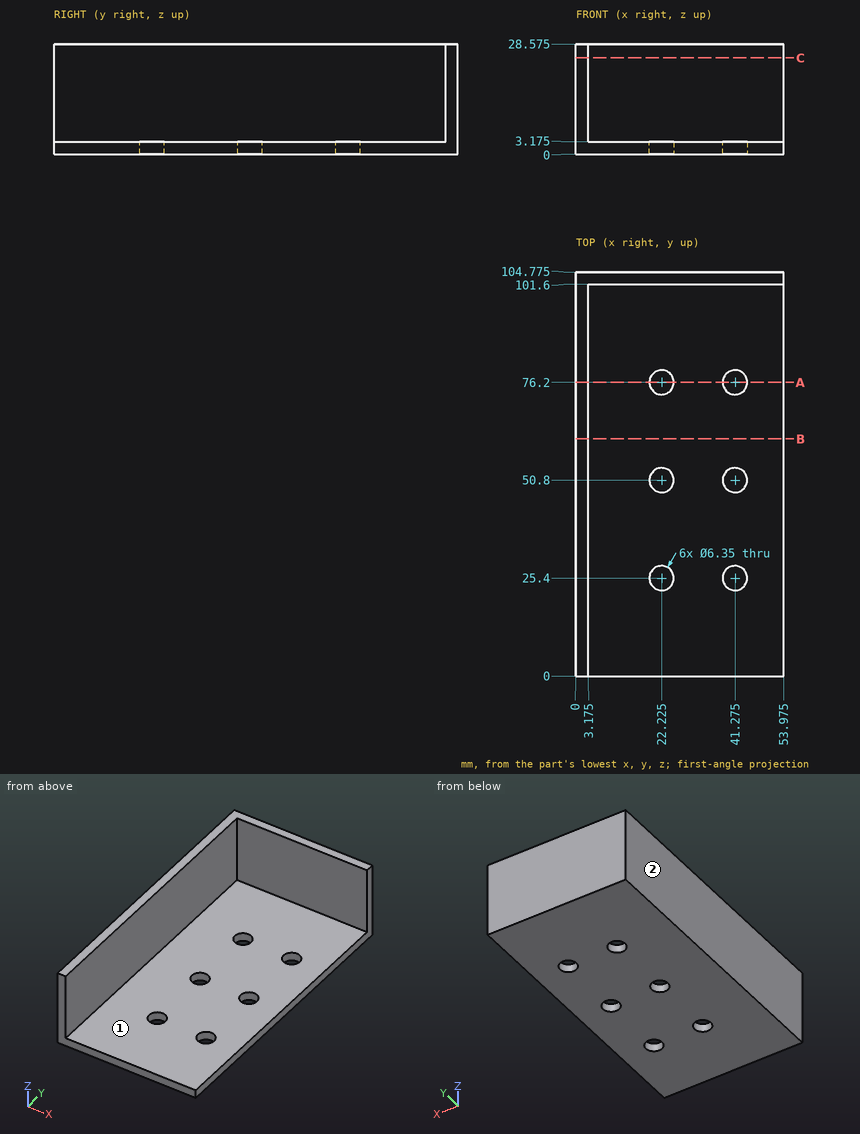
Design review of the part shown in the three views and the two pictorial views. Dimensions are in mm from the part's minimum x, y and z. A direction names the side the tool comes from. Coordinates: 2 decimals unless noted, no trailing zeros. Order: outer loops, then holes, each group sorted by start corner. A loop starts at its lowest first (then second) coordinate and runs counter-clockwise, first axis right, second up. Notation, with made-up numbers: (-16.75, -36.5) -> (8.25, -36.5) arc R18 cw to (8.25, -7.5) -> close; hole circle Ø6 at (85.5, -30). An arc over 180 degrees is marked (long way). Use one line per item in the form item = value. Start each with the question number.
(1) For the marked faces 1 and 2, list the 3-axis set-ups (+Z, -Z, +X, -X, +Y, -Y) from which the entire face can be reached by the end or side of a thin tool; tool diameter is ignored.
(2) Add section A-A on y = 76.2. State the section outline as (x, z) points (3 decimals).
(3) Add section C-C on z = 25. State the section outline as (x, y) points (3 decimals).
(4) Insertion check: pin 1 (6 mm diameter, centred on y = 25, z = 5.5, fed in from -X); pin 2 (1 mm diameter, centred on x = 44.5, z = 23.5, fed in from -Y); pin 3 (8 mm diameter, centred on y = 53, z = 14, fed in from +X) (3 decimals); pin 4 (10 mm diameter, centred on x = 41.275, y = 76.2, fed in from +Z) (3 decimals). Each pin has a flat end and moves straight along its axis. Give the tip position at first contact, or say it passes through.
(5) For probe 1 along Y at (x, z) = (44, 2) (3 decimals); probe 2 along Y at (x, z) = (22, 25) (3 decimals); probe 3 along Z at (x, y) = (9.5, 52) (3 decimals), list the stretches that pass through material, from the lowest coordinate up.
(6) Add section B-B on y = 61.5. State the section outline as (x, z) points (3 decimals), plus the area to 3 significant figures.
Answer block:
q1.face_1 = +Z, +X, -Y
q1.face_2 = +Z, -Z, -X, +Y, -Y
q2.outline = (0, 0) -> (19.05, 0) -> (19.05, 3.175) -> (3.175, 3.175) -> (3.175, 28.575) -> (0, 28.575) -> close; (25.4, 0) -> (38.1, 0) -> (38.1, 3.175) -> (25.4, 3.175) -> close; (44.45, 0) -> (53.975, 0) -> (53.975, 3.175) -> (44.45, 3.175) -> close
q3.outline = (0, 0) -> (3.175, 0) -> (3.175, 101.6) -> (53.975, 101.6) -> (53.975, 104.775) -> (0, 104.775) -> close
q4.pin_1 = 0
q4.pin_2 = 101.6
q4.pin_3 = 3.175
q4.pin_4 = 3.175
q5.probe_1 = 0 to 23.771, 27.029 to 49.171, 52.429 to 74.571, 77.829 to 104.775
q5.probe_2 = 101.6 to 104.775
q5.probe_3 = 0 to 3.175
q6.outline = (0, 0) -> (53.975, 0) -> (53.975, 3.175) -> (3.175, 3.175) -> (3.175, 28.575) -> (0, 28.575) -> close
q6.area = 252 mm²
